```python
from build123d import *

# Parameters (mm, degrees)
F1_DEPTH = 76.2
F3_DEPTH = 63.5
F4_R     = 6.026978
F5_DEPTH = 254


with BuildPart() as f1:
    # F0 (on Front) → F1 (new body)
    with BuildSketch(Plane.XZ):
        Polygon((0, 28.421371), (-38.1, 28.421371), (-38.1, -22.378629), (50.8, -22.378629), align=None)
    extrude(amount=F1_DEPTH)

    # F2 (on face) → F3 (cut)
    with BuildSketch(Plane.XZ.offset(76.2)):
        Polygon((-38.1, 28.421371), (-38.1, 20.109465), (-3.135807, 20.109465), (39.077971, -22.378629), (50.8, -22.378629), (0, 28.421371), align=None)
    extrude(amount=-F3_DEPTH, mode=Mode.SUBTRACT)

    # F4 (on face) → F5 (cut)
    with BuildSketch(Plane(origin=(-38.1, 0, 0), x_dir=(0, -1, 0), z_dir=(-1, 0, 0))):
        with Locations((44.45, -1.134582)):
            Circle(F4_R)
    extrude(amount=-F5_DEPTH, mode=Mode.SUBTRACT)


solid = f1.part
```
Here's how the part is built. I have some questions about the finished solid (model axes, mm). A direction names the side the tool comes from. Coordinates: 2 decimals unless noted, no trailing zeros. Write each loop counter-clockwise with the first axis right and the second up, starting at its lowest first coordinate (ties: lowest second). Pieces come first, ordered by that corner, then holes. Notation, with made-up numbers: M 67.5,-25.75 L 120.5,-25.75 A18 ccw 120.5,-0.75 Z; hole C 5,-15.5 d1. An arc over 180 degrees is marked long. Answer as CSV lines item,"result". Start each with the question number.
Q1. Suppose I cut it at A-A, the plane y = -44.45. List the corners of the cut face in (x, z) for me.
Q2. Suppose I cut it at B-B, the plane x = -20.5. List the corners of the cut face in (y, z) for me, then the cut area to 3 significant figures.
Q3. For faces 5 (the flat face through (-38.1, -38, -2)), 6 (the flat face through (-21, -45, 20.109)), 7 (the flat face through (17.68, -37.84, -0.84)), which set-ups out of +Z, -Z, +X, -X, +Y, -Y let a thin tool reach every point of the face, with its end or its side?
Q4. Suppose I cut it at C-C, the plane z = -18. List the corners of the cut face in (x, y) for me, then the cut area to 3 significant figures.
Q5. I need wall thicknesses on probe 1 along Z at (x, y) = (-16, -44); probe 2 along Z at (x, y) = (-11, -44.45); probe 3 along Z at (x, y) = (-23, -20). Which ranges of each line are inside material? Lowest first, please. Write a range as [from, to].
Q6. If we mould it in two halves opening along Y, with no side actions, what happens to faces 1 (the cylindrical face through (-7.434, -43.143, -7.018)), 2 (the flat face through (-4, 0, -2)), 3 (the flat face through (-19, -6, 28.421)), 4 (the flat face through (-9, -76.2, -6))? For each: pulls with the +Y half, pulls with the -Y half, needs draft (parallel to the pull), parting line crosses it, or undercut.
Q7. Will these pins go through, and if not, where does the flat tip stop? pin 1 Ø8 at (x, y) = (28.5, -34.5) entering from +Z; pin 2 Ø12 at (x, y) = (-20, -53) entering from +Z; pin 3 Ø5 at (y, z) = (-17.5, 7) entering from +X.
Q8. Suppose I cut it at D-D, the plane x = 35.5. List the corners of the cut face in (y, z) for me, then the cut area to 3 significant figures.
Entries:
1,outline,"M -38.1,-22.38 L 39.08,-22.38 L 23.96,-7.16 L -38.1,-7.16 Z; M -38.1,4.89 L 11.98,4.89 L -3.14,20.11 L -38.1,20.11 Z"
2,outline,"M -76.2,-22.38 L 0,-22.38 L 0,28.42 L -12.7,28.42 L -12.7,20.11 L -76.2,20.11 Z; hole C -44.45,-1.13 d12.05"
2,area,"3,230 mm²"
3,face 5,"+Z, -Z, -X, +Y, -Y"
3,face 6,"+Z, +X, -X, -Y"
3,face 7,"+Z, +X, -Y"
4,outline,"M -38.1,-76.2 L 34.73,-76.2 L 34.73,-12.7 L 46.42,-12.7 L 46.42,0 L -38.1,0 Z"
4,area,"5,700 mm²"
5,probe 1,"z = [-22.38, -7.14], [4.88, 20.11]"
5,probe 2,"z = [-22.38, -7.16], [4.89, 20.11]"
5,probe 3,"z = [-22.38, 20.11]"
6,face 1,"undercut"
6,face 2,"pulls with the +Y half"
6,face 3,"needs draft"
6,face 4,"pulls with the -Y half"
7,pin 1,"stops at z = -7.71"
7,pin 2,"stops at z = 20.11"
7,pin 3,"stops at x = 12.37"
8,outline,"M -76.2,-22.38 L 0,-22.38 L 0,-7.08 L -12.7,-7.08 L -12.7,-18.78 L -76.2,-18.78 Z"
8,area,"423 mm²"
